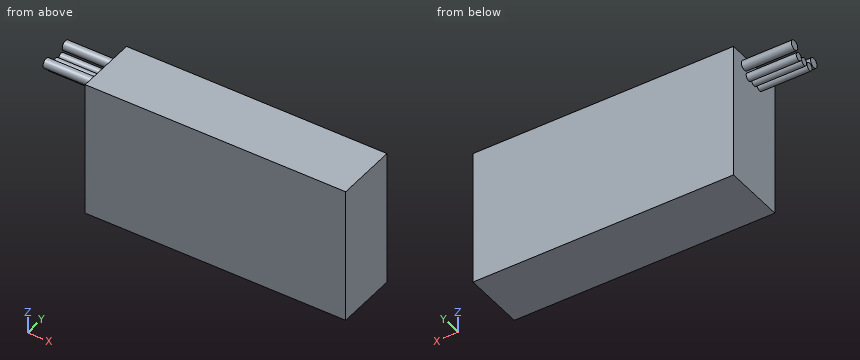
from build123d import *

# Parameters (mm, degrees)
SKETCH1_W           = 67.7
SKETCH1_H           = 16.1
BOSS_EXTRUDE1_DEPTH = 35.3
SKETCH3_R           = 1
SKETCH3_R_2         = 1.25
BOSS_EXTRUDE2_DEPTH = 13


with BuildPart() as part:
    # Sketch1 → Boss-Extrude1 (new body)
    with BuildSketch(Plane.XY):
        with Locations((33.85, 8.05)):
            Rectangle(SKETCH1_W, SKETCH1_H)
    extrude(amount=BOSS_EXTRUDE1_DEPTH)

    # Sketch3 → Boss-Extrude2 (add)
    with BuildSketch(Plane.ZY):
        with Locations(Location((30.7, 10.15, 0), (0, 0, 180))):
            Circle(SKETCH3_R)
        with Locations(Location((30.7, 8.05, 0), (0, 0, 180))):
            Circle(SKETCH3_R)
        with Locations(Location((30.7, 5.95, 0), (0, 0, 180))):
            Circle(SKETCH3_R)
        with Locations(Location((32.8, 4.3, 0), (0, 0, 180))):
            Circle(SKETCH3_R_2)
        with Locations(Location((32.8, 11.8, 0), (0, 0, 180))):
            Circle(SKETCH3_R_2)
    extrude(amount=BOSS_EXTRUDE2_DEPTH)


solid = part.part
The model under review builds one solid part; all positions refer to its coordinate system, in mm. Round coordinates to 2 decimals unless told otherwise and drop trailing zeros. Order: outer loops, then holes, each group sorted by start corner. A loop starts at its lowest first (then second) coordinate and runs counter-clockwise, first axis right, second up. Notation, with made-up numbers: (86.5, 43.5) - (129.5, 43.5) arc R18 ccw to (129.5, 73.5) - close; hole circle Ø11 at (41.25, 6). An arc over 180 degrees is marked (long way). Use one line per item in the form item = value.
Q1. Add section B-B on z = 30.7. Give the boundary of the cut face in (x, y).
Response values:
outline = (-13, 4.95) - (0, 4.95) - (0, 0) - (67.7, 0) - (67.7, 16.1) - (0, 16.1) - (0, 11.15) - (-13, 11.15) - (-13, 9.15) - (0, 9.15) - (0, 9.05) - (-13, 9.05) - (-13, 7.05) - (0, 7.05) - (0, 6.95) - (-13, 6.95) - close
Q2. To check wall thickness, follow line 1 (X direction, y = 12, z = 26); line 2 (Z direction, x = -8.5, y = 12.75). State the ranges of each line that lie inside material, in increasing order.
Response values:
line_1 = 0 to 67.7
line_2 = 31.99 to 33.61
Q3. Add section D-D on z = 17. Give the boundary of the cut face in (x, y), then the cut area to 3 significant figures.
Response values:
outline = (0, 0) - (67.7, 0) - (67.7, 16.1) - (0, 16.1) - close
area = 1,090 mm^2
Q4. Clearance check with a flat-ended pin moving along its axis: P1, Ø1.5, axis at y = 4, z = 18, coming from the -X side. State where the tip first meets the part, or that it passes through.
Response values:
P1 = 0
Q5. Add section C-C on y = 14. Give the boundary of the cut face in (x, z), then the cut area to 3 significant figures.
Response values:
outline = (0, 0) - (67.7, 0) - (67.7, 35.3) - (0, 35.3) - close
area = 2,390 mm^2
Q6. Add section A-A on x = -2. Give the boundary of the cut face in (y, z), then the cut area to 3 significant figures.
Response values:
outline = circle Ø2.5 at (4.3, 32.8); circle Ø2 at (5.95, 30.7); circle Ø2 at (8.05, 30.7); circle Ø2 at (10.15, 30.7); circle Ø2.5 at (11.8, 32.8)
area = 19.2 mm^2
